Work out the finished part from the listing and answer in its coordinate system (mm). Round coordinates to 2 decimals unless told otherwise and drop trailing zeros. Loops run counter-clockwise (first coordinate to the right, second up) from the corner with the lowest first, then second, coordinate; pieces in that order, holes last. Notation, with made-up numbers: (-4.75, -38.75) -> (51.25, -38.75) arc R19 ccw to (51.25, -1.75) -> close; hole circle Ø2 at (63, 48.5). An arc over 180 degrees is marked (long way). Use CSV: the item, a comma, the result in double quotes. Start each with the question number.
from build123d import *

# Parameters (mm, degrees)
F0_R     = 5
F1_DEPTH = 3.175


with BuildPart() as f1:
    # F0 (on Top) → F1 (new body)
    with BuildSketch(Plane.XY):
        with BuildLine():
            Line((-80.835, 25.067168), (-148.335, 25.067168))
            ThreePointArc((-148.335, 25.067168), (-154.835, 18.567168), (-148.335, 12.067168))
            Line((-148.335, 12.067168), (-80.835, 12.067168))
            Line((-80.835, 12.067168), (-13.335, 12.067168))
            Line((-13.335, 12.067168), (54.165, 12.067168))
            Line((54.165, 12.067168), (121.665, 12.067168))
            ThreePointArc((121.665, 12.067168), (128.165, 18.567168), (121.665, 25.067168))
            Line((121.665, 25.067168), (54.165, 25.067168))
            Line((54.165, 25.067168), (-13.335, 25.067168))
            Line((-13.335, 25.067168), (-80.835, 25.067168))
        make_face()
        with Locations((-148.335, 18.567168)):
            Circle(F0_R, mode=Mode.SUBTRACT)
        with Locations((-13.335, 18.567168)):
            Circle(F0_R, mode=Mode.SUBTRACT)
        with Locations((121.665, 18.567168)):
            Circle(F0_R, mode=Mode.SUBTRACT)
    extrude(amount=F1_DEPTH)


solid = f1.part
Q1. Section B-B, the plane y = 16.5 is taken. Write down the section's boundary in (x, z) (3 decimals), and give its area (3 significant figures).
Q2. Section A-A, the plane z = 2.5 is taken. Write down the section's boundary in (x, y) (3 decimals), and give its area (3 significant figures).
Q3. This flat-tipped pin is pushed along its axis until it touches: pin 1 (1.5 mm diameter, centred on y = 16, z = 1.5, fed in from -X). Where does it stop, or does it pass through?
Q4. Straight lines are drawn through the part: line 1 (X direction, y = 19.25, z = 2.6); line 2 (X direction, y = 14.5, z = 2.15); line 3 (X direction, y = 13, z = 2.05). For each, find the intervals that lie inside material, in ascending order. Write a range as from..to.
Q5. For a pull along X with two mould halves and no side action, classify faces 1 (the cylindrical face through (-143.566, 20.069, 1.565)), 2 (the flat face through (-15, 13, 3.175)), 3 (the cylindrical face through (-154.833, 18.71, 1.565)) as pulls with the +X half, pulls with the -X half, needs draft (parallel to the pull), parting line crosses it, or undercut.
Report:
1,outline,"(-154.498, 0) -> (-152.888, 0) -> (-152.888, 3.175) -> (-154.498, 3.175) -> close; (-143.782, 0) -> (-17.888, 0) -> (-17.888, 3.175) -> (-143.782, 3.175) -> close; (-8.782, 0) -> (117.112, 0) -> (117.112, 3.175) -> (-8.782, 3.175) -> close; (126.218, 0) -> (127.828, 0) -> (127.828, 3.175) -> (126.218, 3.175) -> close"
1,area,"810 mm²"
2,outline,"(-148.335, 12.067) -> (121.665, 12.067) arc R6.5 ccw to (121.665, 25.067) -> (-148.335, 25.067) arc R6.5 ccw to start; hole circle Ø10 at (-148.335, 18.567); hole circle Ø10 at (-13.335, 18.567); hole circle Ø10 at (121.665, 18.567)"
2,area,"3,410 mm²"
3,pin 1,"stops at x = -154.58"
4,line 1,"x = -154.8..-153.29, -143.38..-18.29, -8.38..116.71, 126.62..128.13"
4,line 2,"x = -153.41..-151.24, -145.43..-16.24, -10.43..118.76, 124.57..126.74"
4,line 3,"x = -151.69..125.02"
5,face 1,"undercut"
5,face 2,"needs draft"
5,face 3,"pulls with the -X half"
